Read the model definition and answer for the solid it produces. Units are mm, in the model's axes. A direction names the side the tool comes from. Coordinates: 2 decimals unless noted, no trailing zeros. Loops run counter-clockwise (first coordinate to the right, second up) from the corner with the lowest first, then second, coordinate; pieces in that order, holes last.
from build123d import *

# Parameters (mm, degrees)
F0_W     = 279.4
F0_H     = 203.2
F1_DEPTH = 203.2
F5_W     = 228.6
F5_H     = 152.4
F6_DEPTH = 152.4
F2_R     = 6.35
F7_DEPTH = 25.4
F3_R     = 6.35
F8_DEPTH = 25.4
F4_R     = 6.35
F9_DEPTH = 25.4


with BuildPart() as f1:
    # F0 (on Front) → F1 (new body)
    with BuildSketch(Plane.XZ):
        Rectangle(F0_W, F0_H)
    extrude(amount=-F1_DEPTH)

    # F5 (on Front) → F6 (cut)
    with BuildSketch(Plane.XZ):
        Rectangle(F5_W, F5_H)
    extrude(amount=-F6_DEPTH, mode=Mode.SUBTRACT)

    # F2 (on face) → F7 (cut)
    with BuildSketch(Plane.XY.offset(101.6)):
        with Locations((0, 101.6)):
            Circle(F2_R)
    extrude(amount=-F7_DEPTH, mode=Mode.SUBTRACT)

    # F3 (on face) → F8 (cut)
    with BuildSketch(Plane.YZ.offset(139.7)):
        with Locations((101.6, 0)):
            Circle(F3_R)
    extrude(amount=-F8_DEPTH, mode=Mode.SUBTRACT)

    # F4 (on face) → F9 (cut)
    with BuildSketch(Plane(origin=(-139.7, 0, 0), x_dir=(0, -1, 0), z_dir=(-1, 0, 0))):
        with Locations((-101.6, 0)):
            Circle(F4_R)
    extrude(amount=-F9_DEPTH, mode=Mode.SUBTRACT)


solid = f1.part
Q1. A cutting plane is placed at A-A (x = 0). Give the vertices of the cut face in (y, z), then the cut area to 3 significant figures.
Findings below:
outline: (0, -101.6) - (203.2, -101.6) - (203.2, 101.6) - (107.95, 101.6) - (107.95, 76.2) - (152.4, 76.2) - (152.4, -76.2) - (0, -76.2) - close; (0, 76.2) - (95.25, 76.2) - (95.25, 101.6) - (0, 101.6) - close
area: 17,700 mm2
Q2. A cutting plane is placed at D-D (y = 53.5). Give the vertices of the cut face in (x, z).
Findings below:
outline: (-139.7, -101.6) - (139.7, -101.6) - (139.7, 101.6) - (-139.7, 101.6) - close; hole (-114.3, -76.2) - (114.3, -76.2) - (114.3, 76.2) - (-114.3, 76.2) - close
Q3. A cutting plane is placed at C-C (y = 101.6). Give the vertices of the cut face in (x, z).
Findings below:
outline: (-139.7, -101.6) - (139.7, -101.6) - (139.7, -6.35) - (114.3, -6.35) - (114.3, -76.2) - (-114.3, -76.2) - (-114.3, -6.35) - (-139.7, -6.35) - close; (-139.7, 6.35) - (-114.3, 6.35) - (-114.3, 76.2) - (-6.35, 76.2) - (-6.35, 101.6) - (-139.7, 101.6) - close; (6.35, 76.2) - (114.3, 76.2) - (114.3, 6.35) - (139.7, 6.35) - (139.7, 101.6) - (6.35, 101.6) - close
Q4. Straight lines are drawn through the part: probe 1 along X at (y, z) = (90.5, -76); probe 2 along Z at (x, y) = (123.75, 101.6); probe 3 along Z at (x, y) = (-54.5, 64). For each, find the intervals that lie inside material, in ascending order.
Findings below:
probe 1: x = -139.7 to -114.3, 114.3 to 139.7
probe 2: z = -101.6 to -6.35, 6.35 to 101.6
probe 3: z = -101.6 to -76.2, 76.2 to 101.6
Q5. A cutting plane is placed at B-B (z = 0). Give the vertices of the cut face in (x, y).
Findings below:
outline: (-139.7, 0) - (-114.3, 0) - (-114.3, 95.25) - (-139.7, 95.25) - close; (-139.7, 107.95) - (-114.3, 107.95) - (-114.3, 152.4) - (114.3, 152.4) - (114.3, 107.95) - (139.7, 107.95) - (139.7, 203.2) - (-139.7, 203.2) - close; (114.3, 0) - (139.7, 0) - (139.7, 95.25) - (114.3, 95.25) - close
Q6. Determine the mould class of faces 4 (the face through (127.178, 107.657, 1.907)), 5 (the face through (-2, 203.2, 1)), 6 (the face through (-114.3, 75, -1)) for opening direction Y: +Y half, -Y half, draft (parallel to the pull), parting line (faces both ways), or undercut.
Findings below:
face 4: undercut
face 5: +Y half
face 6: draft
Q7. Which of the six approach directions +Z, -Z, +X, -X, +Y, -Y give full straight-line access (tool end or side, diameter ignored) to faces 1 (the face through (-0.8, 107.9, 89.1)), 2 (the face through (-127.178, 107.944, 0.279)), 3 (the face through (-2, 75, 76.2))?
Findings below:
face 1: +Z
face 2: +X, -X
face 3: -Y
